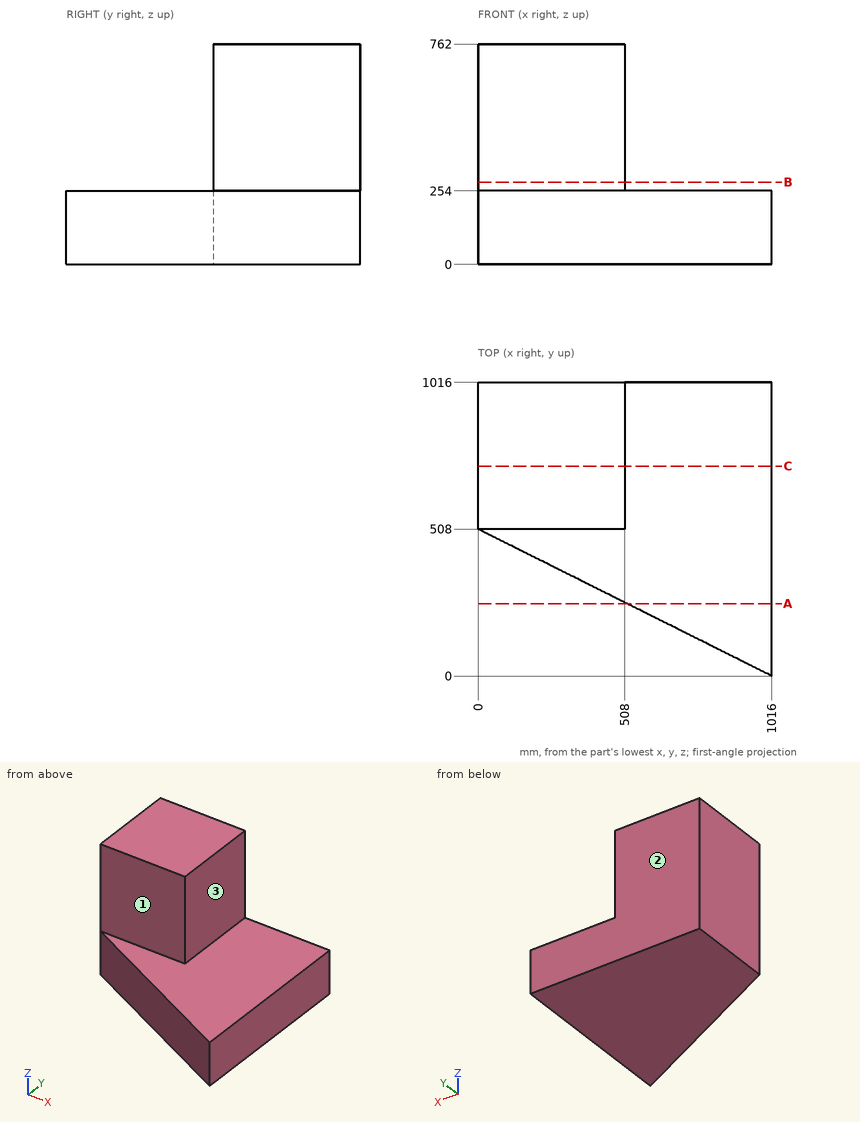
Here's the drawing with two shaded views (mm, measured from the low corner). I have some questions. A direction names the side the tool comes from. Give positions to 0.01 mm unless a question says otherwise; leave off trailing zeros. Order: outer loops, then holes, each group sorted by start corner. A loop starts at its lowest first (then second) coordinate and runs counter-clockwise, first axis right, second up.
Q1. Suppose I cut it at B-B, the plane z = 284.5. Write out the boundary of the cut face in (x, y), and give its area (3 significant figures).
Q2. Suppose I cut it at A-A, the plane y = 250. Write out the boundary of the cut face in (x, z).
Q3. I'm going to push flat-ended pins straight in: P1, Ø3, axis at x = 649, z = 247.5, coming from the -Y side; P2, Ø3, axis at x = 322.5, z = 678, coming from the -Y side; P3, Ø12, axis at y = 536.5, z = 550, coming from the +X side. Where does each tip first touch, or does it pass through?
Q4. For the marked faces 1, 2 and 3, which set-ups out of +Z, -Z, +X, -X, +Y, -Y let a thin tool reach every point of the face, with its end or its side?
Q5. Suppose I cut it at C-C, the plane y = 726. Write out the boundary of the cut face in (x, z), and give its area (3 significant figures).
Q6. If I drill on line 1 along X through (y, z) = (806, 613.5); line 2 along Y through (x, z) = (120.5, 365); line 3 along Z through (x, y) = (540, 325), over which ranges is the centre line in solid material (lowest first)?
Solution:
1. outline: (0, 508) - (508, 508) - (508, 1016) - (0, 1016) - close
1. area: 258,000 mm2
2. outline: (516, 0) - (1016, 0) - (1016, 254) - (516, 254) - close
3. P1: stops at y = 182.75
3. P2: stops at y = 508
3. P3: stops at x = 508
4. face 1: +Z, +X, -X, -Y
4. face 2: +Z, -Z, +X, -X, +Y
4. face 3: +Z, +X, +Y, -Y
5. outline: (0, 0) - (1016, 0) - (1016, 254) - (508, 254) - (508, 762) - (0, 762) - close
5. area: 516,000 mm2
6. line 1: x = 0 to 508
6. line 2: y = 508 to 1016
6. line 3: z = 0 to 254
